```python
from build123d import *

# Parameters (mm, degrees)
F0_W     = 13.378338
F0_H     = 10.662744
F1_DEPTH = 4.57033
F2_R     = 3.578427
F3_DEPTH = 3.60733
F4_R     = 5.08


with BuildPart() as f1:
    # F0 (on Front) → F1 (new body)
    with BuildSketch(Plane.XZ):
        with Locations((-3.845378, 0.310359)):
            Rectangle(F0_W, F0_H)
    extrude(amount=F1_DEPTH)

    # F2 (on face) → F3 (cut)
    with BuildSketch(Plane.XZ.offset(4.57033)):
        with Locations((-4.26886, 0)):
            Circle(F2_R)
    extrude(amount=-F3_DEPTH, mode=Mode.SUBTRACT)

    # F4
    f4_edges = [f1.edges().sort_by_distance(p)[0] for p in [
        (2.843791, -2.285165, -5.021013),
        (2.843791, -2.285165, 5.641731),
        (-10.534547, -2.285165, 5.641731),
        (-10.534547, -2.285165, -5.021013),
    ]]
    fillet(f4_edges, radius=F4_R)


solid = f1.part
```
Input: part model. Units: mm. Frame: model coordinates. A direction names the side the tool comes from. Round coordinates to 2 decimals unless told otherwise and drop trailing zeros. Order: outer loops, then holes, each group sorted by start corner. A loop starts at its lowest first (then second) coordinate and runs counter-clockwise, first axis right, second up. Notation, with made-up numbers: (13.25, -12.5) - (72.25, -12.5) arc R27 ccw to (72.25, 24.5) - close; hole circle Ø1 at (-3, 43). An arc over 180 degrees is marked (long way). One line per question, with ' | ' between items. Start each with the question number.
1) Contact query for a flat-ended pin moving along its axis: P1, Ø4.5, axis at x = -4.27, z = 0, coming from the -Y side. Output: stop coordinate, or through.
2) Ray query, probe 1 along Y at (x, z) = (-3, 2); probe 2 along X at (y, z) = (-2.3, -0.75); probe 3 along Z at (x, y) = (-5.5, -2.15). Return the intervals inside material, ascending.
3) Cut plane B-B, the plane x = -2. Return the cut outline in (y, z).
4) Cut plane C-C, the plane x = -5. Return the cut outline in (y, z), then the cut area to 3 significant figures.
5) Pull-direction query (Z, two-part tool) for faces 3 (the flat face through (-4, -0.963, 0)), 4 (the cylindrical face through (-9.1, -2.3, 4.1)), 5 (the flat face through (-4, 0, 0)), 6 (the cylindrical face through (-9.09, -2.32, -3.49)); classes: +Z half, -Z half, draft (parallel to the pull), parting line (faces both ways), or undercut.
6) Cut plane A-A, the plane y = -2.75. Return the cut outline in (x, z).
7) Cut plane D-D, the plane x = 0.5. Return the cut outline in (y, z), then the cut area to 3 significant figures.
8) Set-up query: faces 1 (the cylindrical face through (1.32, -2.32, 4.19)), 2 (the cylindrical face through (-0.856, -2.792, 1.075)). Return all of +Z, -Z, +X, -X, +Y, -Y with unobstructed straight access to the full face (end or side cutting, diameter ignored); none if empty.
Worked out:
1) P1: stops at y = -0.96
2) probe 1: y = -0.96 to 0 | probe 2: x = -10.47 to -7.77, -0.77 to 2.78 | probe 3: z = -5.02 to -3.36, 3.36 to 5.64
3) outline: (-4.57, -5.02) - (0, -5.02) - (0, 5.64) - (-4.57, 5.64) - (-4.57, 2.77) - (-0.96, 2.77) - (-0.96, -2.77) - (-4.57, -2.77) - close
4) outline: (-4.57, -5.02) - (0, -5.02) - (0, 5.64) - (-4.57, 5.64) - (-4.57, 3.5) - (-0.96, 3.5) - (-0.96, -3.5) - (-4.57, -3.5) - close | area: 23.5 mm^2
5) face 3: undercut | face 4: +Z half | face 5: draft | face 6: -Z half
6) outline: (-10.53, 0.06) arc R5.08 ccw to (-5.45, -5.02) - (-2.24, -5.02) arc R5.08 ccw to (2.84, 0.06) - (2.84, 0.56) arc R5.08 ccw to (-2.24, 5.64) - (-5.45, 5.64) arc R5.08 ccw to (-10.53, 0.56) - close; hole circle Ø7.16 at (-4.27, 0)
7) outline: (-4.57, -4.22) - (0, -4.22) - (0, 4.84) - (-4.57, 4.84) - close | area: 41.4 mm^2
8) face 1: +Z, +X, +Y, -Y | face 2: -Y
